Geometry check sheet. Reference: the model listing, model coordinates, mm. A direction names the side the tool comes from. Round coordinates to 2 decimals unless told otherwise and drop trailing zeros. Loops run counter-clockwise (first coordinate to the right, second up) from the corner with the lowest first, then second, coordinate; pieces in that order, holes last. Notation, with made-up numbers: (46, 58.25) -> (97, 58.25) arc R25 ccw to (97, 74.25) -> close; hole circle Ø5 at (70.5, 15). An arc over 180 degrees is marked (long way). Use a Markdown table: item, result. Add a question column.
Q1. Sectioned sample at A-A, the plane x = 3. Enter the section's corners in (y, z).
Q2. Sectioned sample at B-B, the plane y = 27.13. Enter the section's corners in (x, z).
Q3. Material ranges on L1, parallel to Y at x = 27, z = 0.85; L2, parallel to Y at x = 17.5, z = 2.4, recorded low to high.
Q4. Sectioned sample at C-C, the plane y = 12. Enter the section's corners in (x, z).
Q5. Gauge pin test, flat ends, axial feed: P1, Ø1.8, axis at y = 12.5, z = 2.5, coming from the +X side; P2, Ø4, axis at x = 3, y = 2.87, coming from the +Z side; P3, Ø3, axis at x = 27, y = 27.13, coming from the -Z side; P4, Ø1.8, axis at x = 16.5, z = 3.5, coming from the -Y side. Record the tip position at first contact, or that the pin passes through.
Q6. Release check for a two-part mould opening along Y. For faces 5 (the face through (15, 15, 5)), 6 (the face through (0.376, 0.356, 0.493)), 7 (the face through (25.7, 3.8, 0.5)) record: released by +Y, released by -Y, zero draft, split by the parting line, or undercut.
Q7. Set-up check for faces 1 (the face through (21, 15, 3)), 2 (the face through (15, 9, 3)), 3 (the face through (9, 15, 3)), 4 (the face through (14.8, 30, 0.5)): record each of +Z, -Z, +X, -X, +Y, -Y from which the full face is reachable in a straight line by a thin tool's end or side.
Autodesk Fusion 360 part; units mm, degrees
sketch "スケッチ1" plane through (0, 0, 0) normal (0, 0, 1) x (1, 0, 0)
  line L0 (0, 0) -> (30, 0)
  line L1 (30, 0) -> (0, 0)
  line L2 (0, 0) -> (0, 30)
  line L3 (0, 30) -> (30, 30)
  line L4 (30, 30) -> (30, 0)
  line L5 (0, 0) -> (1.25, 0)
  line L6 (0, 0) -> (0, 1.25)
  arc A0 (0, 1.25) -> (1.25, 0) centre (1.25, 1.25) ccw
  arc A1 (1.25, 30) -> (0, 28.75) centre (1.25, 28.75) ccw
  arc A2 (30, 28.75) -> (28.75, 30) centre (28.75, 28.75) ccw
  arc A3 (28.75, 0) -> (30, 1.25) centre (28.75, 1.25) ccw
  line L7 (0, 30) -> (0, 28.73)
  circle A4 centre (3, 27.13) radius 1.6
  circle A5 centre (27, 27.13) radius 1.6
  circle A6 centre (27, 2.87) radius 1.6
  circle A7 centre (3, 2.87) radius 1.6
  dimension "d1" = 30
  dimension "d2" = 1.25
  dimension "d3" = 1.25
  dimension "d4" = 1.27
  dimension "d6" = 3.2
extrude "押し出し1" add sketch "スケッチ1" along normal blind 1 contours L0 L1 L2 L3 L4 A0 A1 A2 A3 L7
sketch "スケッチ2" plane through (0, 0, 1) normal (0, 0, 1) x (-1, 0, 0)
  circle A0 centre (-3, -27.13) radius 1.6
  circle A1 centre (-3, -2.87) radius 1.6
  circle A2 centre (-27, -2.87) radius 1.6
  circle A3 centre (-27, -27.13) radius 1.6
  arc A4 (-30, -28.75) -> (-28.75, -30) centre (-28.75, -28.75) ccw
  line L0 (-28.75, -30) -> (-1.25, -30)
  arc A5 (-1.25, -30) -> (0, -28.75) centre (-1.25, -28.75) ccw
  line L1 (0, -28.75) -> (0, -1.25)
  arc A6 (0, -1.25) -> (-1.25, 0) centre (-1.25, -1.25) ccw
  line L2 (-1.25, 0) -> (-28.75, 0)
  arc A7 (-28.75, 0) -> (-30, -1.25) centre (-28.75, -1.25) ccw
  line L3 (-30, -1.25) -> (-30, -28.75)
  line L4 (-8, -22) -> (-8, -8)
  line L5 (-8, -8) -> (-22, -8)
  line L6 (-22, -8) -> (-22, -22)
  line L7 (-22, -22) -> (-8, -22)
sketch "スケッチ3" plane through (0, 0, 1) normal (0, 0, 1) x (-1, 0, 0)
  circle A0 centre (-3, -27.13) radius 1.6
  circle A1 centre (-3, -2.87) radius 1.6
  circle A2 centre (-27, -2.87) radius 1.6
  circle A3 centre (-27, -27.13) radius 1.6
  arc A4 (-30, -28.75) -> (-28.75, -30) centre (-28.75, -28.75) ccw
  line L0 (-28.75, -30) -> (-1.25, -30)
  arc A5 (-1.25, -30) -> (0, -28.75) centre (-1.25, -28.75) ccw
  line L1 (0, -28.75) -> (0, -1.25)
  arc A6 (0, -1.25) -> (-1.25, 0) centre (-1.25, -1.25) ccw
  line L2 (-1.25, 0) -> (-28.75, 0)
  arc A7 (-28.75, 0) -> (-30, -1.25) centre (-28.75, -1.25) ccw
  line L3 (-30, -1.25) -> (-30, -28.75)
  line L4 (-9, -21) -> (-9, -9)
  line L5 (-9, -9) -> (-21, -9)
  line L6 (-21, -9) -> (-21, -21)
  line L7 (-21, -21) -> (-9, -21)
extrude "押し出し3" add sketch "スケッチ3" along normal blind 4 contours L4 L5 L6 L7
fillet "フィレット2" radius 0.5 1 faces at (13, 17, 5)
extrude "押し出し2" [suppressed]
fillet "フィレット1" [suppressed]
Values:
| question | item | result |
|---|---|---|
| 1 | outline | (0, 0) -> (1.27, 0) -> (1.27, 1) -> (0, 1) -> close; (4.47, 0) -> (25.53, 0) -> (25.53, 1) -> (4.47, 1) -> close; (28.73, 0) -> (30, 0) -> (30, 1) -> (28.73, 1) -> close |
| 2 | outline | (0, 0) -> (1.4, 0) -> (1.4, 1) -> (0, 1) -> close; (4.6, 0) -> (25.4, 0) -> (25.4, 1) -> (4.6, 1) -> close; (28.6, 0) -> (30, 0) -> (30, 1) -> (28.6, 1) -> close |
| 3 | L1 | 0 to 1.27, 4.47 to 25.53, 28.73 to 30 |
| 3 | L2 | 9 to 21 |
| 4 | outline | (0, 0) -> (30, 0) -> (30, 1) -> (21, 1) -> (21, 4.5) arc R0.5 ccw to (20.5, 5) -> (9.5, 5) arc R0.5 ccw to (9, 4.5) -> (9, 1) -> (0, 1) -> close |
| 5 | P1 | x = 21 |
| 5 | P2 | z = 1 |
| 5 | P3 | through |
| 5 | P4 | y = 9 |
| 6 | face 5 | zero draft |
| 6 | face 6 | released by -Y |
| 6 | face 7 | undercut |
| 7 | face 1 | +Z, +X, +Y, -Y |
| 7 | face 2 | +Z, +X, -X, -Y |
| 7 | face 3 | +Z, -X, +Y, -Y |
| 7 | face 4 | +Z, -Z, +X, -X, +Y |
